Autodesk Inventor part; units mm, degrees
ref_plane "YZ Plane" through (0, 0, 0) normal (1, 0, 0) x (0, 1, 0)
ref_plane "XZ Plane" through (0, 0, 0) normal (0, 1, 0) x (-1, 0, 0)
ref_plane "XY Plane" through (0, 0, 0) normal (0, 0, 1) x (1, 0, 0)
sketch "Sketch1" plane through (0, 0, 0) normal (0, 0, 1) x (1, 0, 0)
  line L0 (-4, 0) -> (-194, 0)
  line L1 (-198, 4) -> (-198, 27)
  line L2 (-194, 31) -> (-4, 31)
  line L3 (0, 27) -> (0, 4)
  arc A0 (0, 27) -> (-4, 31) centre (-4, 27) ccw
  arc A1 (-194, 31) -> (-198, 27) centre (-194, 27) ccw
  arc A2 (-198, 4) -> (-194, 0) centre (-194, 4) ccw
  arc A3 (-4, 0) -> (0, 4) centre (-4, 4) ccw
  point P0 (0, 0)
  point P1 (-198, 0)
  point P2 (0, 31)
  dimension "d0" = 198
  dimension "d1" = 31
  dimension "d2" = 4
extrude "Extrusion1" add sketch "Sketch1" along normal blind 2
sketch "Sketch2" plane through (0, 0, 0) normal (0, 0, -1) x (-1, 0, 0)
  line L0 (95.9784, 21.4874) -> (112.8534, 21.4874)
  line L1 (112.8534, 21.4874) -> (112.8534, 7)
  line L2 (112.8534, 7) -> (95.9784, 7)
  line L3 (95.9784, 7) -> (95.9784, 21.4874)
  line L4 (194, 0) -> (4, 0)
  line L5 (0, 4) -> (0, 27)
  line L6 (115.1046, 23.6) -> (131.2046, 23.6)
  line L7 (131.2046, 23.6) -> (131.2046, 7)
  line L8 (131.2046, 7) -> (115.1046, 7)
  line L9 (115.1046, 7) -> (115.1046, 23.6)
  line L10 (133.1046, 23.6) -> (149.2046, 23.6)
  line L11 (149.2046, 23.6) -> (149.2046, 7)
  line L12 (149.2046, 7) -> (133.1046, 7)
  line L13 (133.1046, 7) -> (133.1046, 23.6)
  circle A0 centre (162.7, 14.5) radius 3.5
  circle A1 centre (178, 14.5) radius 3.5
  line L14 (198, 27) -> (198, 4)
  line L15 (70.05, 15.74) -> (56.95, 15.74)
  line L16 (56.95, 15.74) -> (56.95, 27.6)
  line L17 (56.95, 27.6) -> (70.05, 27.6)
  line L18 (70.05, 27.6) -> (70.05, 15.74)
  circle A2 centre (77, 21.67) radius 3
  circle A3 centre (50, 21.67) radius 3
  line L19 (63.5, 15.74) -> (63.5, 8.0383)
  line L20 (32.5145, 26.3095) -> (17.7855, 26.3095)
  line L21 (15.7855, 24.3095) -> (15.7855, 20.8274)
  line L22 (17.1974, 18.9158) -> (17.2455, 18.901)
  line L23 (18.1588, 18.3108) -> (18.6882, 17.7092)
  line L24 (20.1896, 17.0305) -> (30.1104, 17.0305)
  line L25 (31.6118, 17.7092) -> (32.1412, 18.3108)
  line L26 (33.0545, 18.901) -> (33.1026, 18.9158)
  line L27 (34.5145, 20.8274) -> (34.5145, 24.3095)
  circle A4 centre (38.3, 21.67) radius 1.75
  circle A5 centre (12, 21.67) radius 1.75
  arc A6 (33.1026, 18.9158) -> (34.5145, 20.8274) centre (32.5145, 20.8274) ccw
  arc A7 (33.0545, 18.901) -> (32.1412, 18.3108) centre (33.6426, 16.9895) ccw
  arc A8 (30.1104, 17.0305) -> (31.6118, 17.7092) centre (30.1104, 19.0305) ccw
  arc A9 (18.6882, 17.7092) -> (20.1896, 17.0305) centre (20.1896, 19.0305) ccw
  arc A10 (18.1588, 18.3108) -> (17.2455, 18.901) centre (16.6574, 16.9895) ccw
  arc A11 (15.7855, 20.8274) -> (17.1974, 18.9158) centre (17.7855, 20.8274) ccw
  arc A12 (17.7855, 26.3095) -> (15.7855, 24.3095) centre (17.7855, 24.3095) ccw
  arc A13 (34.5145, 24.3095) -> (32.5145, 26.3095) centre (32.5145, 24.3095) ccw
  point P0 (0, 0)
  point P1 (34.5145, 26.3095)
  point P2 (15.7855, 26.3095)
  point P3 (15.7855, 19.3502)
  point P4 (17.7855, 18.7349)
  point P5 (19.2855, 17.0305)
  point P6 (31.0145, 17.0305)
  point P7 (32.5145, 18.7349)
  point P8 (34.5145, 19.3502)
  dimension "d7" = 16.875
  dimension "d8" = 14.4874
  dimension "d9" = 7
  dimension "d11" = 2.2512
  dimension "d12" = 1.9
  dimension "d13" = 16.1
  dimension "d14" = 16.1
  dimension "d15" = 16.6
  dimension "d16" = 7
  dimension "d17" = 7
  dimension "d18" = 7.5
  dimension "d19" = 13.4954
  dimension "d20" = 15.3
  dimension "d21" = 20
  dimension "d22" = 13.1
  dimension "d23" = 11.86
  dimension "d26" = 27
  dimension "d27" = 6
  dimension "d28" = 13.5
  dimension "d29" = 5.93
  dimension "d30" = 9.279
  dimension "d31" = 18.729
  dimension "d32" = 107.1
  dimension "d33" = 107.1
  dimension "d34" = 138.65
  dimension "d35" = 138.65
  dimension "d36" = 2
  dimension "d37" = 2
  dimension "d38" = 3.5
  dimension "d39" = 3.5
  dimension "d40" = 3.5
  dimension "d41" = 26.3
  dimension "d42" = 3.7855
  dimension "d43" = 4.6395
  dimension "d45" = 2
  dimension "d47" = 50
  dimension "d48" = 12
  dimension "d49" = 4
extrude "Extrusion2" cut sketch "Sketch2" against normal through all
equation "\"d2\" = filletMid"
equation "\"d3\" = thickness"
equation "\"d14\" = d13"
equation "\"d21\" = offsetFromSideOfCase"
equation "\"d28\" = 0.5 * d26"
equation "\"d29\" = 0.5 * d23"
equation "\"d33\" = d32"
equation "\"d35\" = d34"
equation "\"d42\" = -0.5 * d31 + 0.5 * d41"
equation "\"d43\" = 0.5 * d30"
equation "\"d5\" = thickness"
properties part number "case-back"
CAD build for the part. Positions are in the model's coordinates, mm. Coordinates: 2 decimals unless noted, no trailing zeros. Order: outer loops, then holes, each group sorted by start corner. A loop starts at its lowest first (then second) coordinate and runs counter-clockwise, first axis right, second up. Notation, with made-up numbers: (-27, 18) - (-8, 18) arc R32 cw to (-8, 50) - close; hole circle Ø3 at (-32.75, 19). An arc over 180 degrees is marked (long way). Use a Markdown table: item, result. Add a question column.
(1) Saw through at A-A (y = 9). Give the cut face in (x, z).
(2) Pull direction X, two halves, no side cores. Call faces 1 (the face through (-47.003, 21.802, 0.986)), 2 (the face through (-100, 23, 0)), 3 (the face through (-1.203, 29.859, 0.986)): +X half, -X half, draft (parallel to the pull), parting line (faces both ways), or undercut.
(3) Drill centre lines: line 1 along X through (y, z) = (15, 0.7); line 2 along X through (y, z) = (9, 1.2); line 3 along Y through (x, z) = (-105.5, 1.4). Where is each one in solid material? Low to high. Write a range as [from, to].
(4) Saw through at D-D (z = 0.6). Count the separate pieces of the cut face and the enclosed holes in it, then the cut area to 3 significant figures.
(5) Saw through at B-B (x = -77). Give the cut face in (y, z), then the cut area to 3 significant figures.
(6) Saw through at C-C (x = -141.5). Give the cut face in (y, z).
Solved:
| question | item | result |
|---|---|---|
| 1 | outline | (-198, 0) - (-149.2, 0) - (-149.2, 2) - (-198, 2) - close; (-133.1, 0) - (-131.2, 0) - (-131.2, 2) - (-133.1, 2) - close; (-115.1, 0) - (-112.85, 0) - (-112.85, 2) - (-115.1, 2) - close; (-95.98, 0) - (0, 0) - (0, 2) - (-95.98, 2) - close |
| 2 | face 1 | undercut |
| 2 | face 2 | draft |
| 2 | face 3 | +X half |
| 3 | line 1 | x = [-198, -181.46], [-174.54, -166.16], [-159.24, -149.2], [-133.1, -131.2], [-115.1, -112.85], [-95.98, 0] |
| 3 | line 2 | x = [-198, -149.2], [-133.1, -131.2], [-115.1, -112.85], [-95.98, 0] |
| 3 | line 3 | y = [0, 7], [21.49, 31] |
| 4 | separate pieces | 1 |
| 4 | enclosed holes | 11 |
| 4 | area | 4,880 mm² |
| 5 | outline | (0, 0) - (18.67, 0) - (18.67, 2) - (0, 2) - close; (24.67, 0) - (31, 0) - (31, 2) - (24.67, 2) - close |
| 5 | area | 50.0 mm² |
| 6 | outline | (0, 0) - (7, 0) - (7, 2) - (0, 2) - close; (23.6, 0) - (31, 0) - (31, 2) - (23.6, 2) - close |
